Autodesk Inventor part; units mm, degrees
ref_plane "YZ Plane" through (0, 0, 0) normal (1, 0, 0) x (0, 1, 0)
ref_plane "XZ Plane" through (0, 0, 0) normal (0, 1, 0) x (-1, 0, 0)
ref_plane "XY Plane" through (0, 0, 0) normal (0, 0, 1) x (1, 0, 0)
sketch "Sketch1" plane through (0, 0, 0) normal (0, 0, 1) x (1, 0, 0)
  line L0 (-81.3375, 50) -> (81.3375, 50)
  line L1 (81.3375, 50) -> (81.3375, -50)
  line L2 (81.3375, -50) -> (-81.3375, -50)
  line L3 (-81.3375, -50) -> (-81.3375, 50)
  point P0 (0, 0)
  point P1 (0, 50)
  point P2 (81.3375, 0)
  dimension "d0" = 100
  dimension "d1" = 162.675
extrude "Extrusion1" add sketch "Sketch1" along normal blind 10
sketch "Sketch2" plane through (0, 0, 10) normal (0, 0, 1) x (1, 0, 0)
  line L0 (10.6002, 14) -> (68.6002, 14) construction
  line L1 (68.6002, 14) -> (68.6002, -35) construction
  line L2 (68.6002, -35) -> (10.6002, -35) construction
  line L3 (10.6002, -35) -> (10.6002, 14) construction
  line L4 (-81.3375, -50) -> (81.3375, -50)
  point P0 (0, 0)
  dimension "d4" = 58
  dimension "d5" = 49
  dimension "d18" = 15
hole "Hole1" at (10.6002, 14, 10) at (68.6002, 14, 10) at (68.6002, -35, 10) at (10.6002, -35, 10) direction (0, 0, -1) diameter 3 end through all
sketch "Sketch3" plane through (0, 0, 10) normal (0, 0, 1) x (1, 0, 0)
  line L0 (14.1002, -32.35) -> (65.1002, -32.35)
  line L1 (65.1002, -32.35) -> (65.1002, -37.65)
  line L2 (65.1002, -37.65) -> (14.1002, -37.65)
  line L3 (14.1002, -37.65) -> (14.1002, -32.35)
  circle A0 centre (68.6002, -35) radius 1.5
  circle A1 centre (10.6002, -35) radius 1.5
  line L4 (10.6002, -35) -> (68.6002, -35) construction
  point P0 (0, 0)
  point P1 (65.1002, -35)
  point P2 (39.6002, -35)
  point P3 (39.6002, -32.35)
  dimension "d14" = 5.3
  dimension "d15" = 51
extrude "Extrusion2" cut sketch "Sketch3" against normal through all contours L0 L1 L2 L3
mirror "Mirror1" about plane through (0, 0, 0) normal (1, 0, 0) of "Hole1", "Extrusion2"
fillet "Fillet1" radius 3 4 edges at (81.3375, 50, 5) (-81.3375, 50, 5) (-81.3375, -50, 5) (81.3375, -50, 5)
equation "\"d1\" = 2.5 * width"
equation "\"hight\" = 56.21"
equation "\"width\" = 65.07"
properties part number "RasPi-Hat-outline"
Can you work these out from the model? Positions are in its coordinate system, mm. A direction names the side the tool comes from. Give positions to 0.01 mm unless a question says otherwise; leave off trailing zeros. Loops run counter-clockwise (first coordinate to the right, second up) from the corner with the lowest first, then second, coordinate; pieces in that order, holes last. Notation, with made-up numbers: (80, 46) - (100, 46) arc R9 cw to (100, 51) - close; hole circle Ø7 at (48, -37.75). An arc over 180 degrees is marked (long way). One line per item, written item: value.
(1) If we mould it in two halves opening along Y, with no side actions, what happens to faces 3 (the face through (-9.7, -33.8, 4.9)), 4 (the face through (-1, 1, 0)), 5 (the face through (80.48, 49.1, 5.07))? For each: released by +Y, released by -Y, zero draft, split by the parting line, or undercut.
Verdict:
face 3: undercut
face 4: zero draft
face 5: released by +Y
(2) I need wall thicknesses on line 1 along X through (y, z) = (14, 8); line 2 along Y through (x, z) = (48.5, 1.75). Which ranges of each line are inside material? Lowest first, please.
Verdict:
line 1: -81.34 to -70.1, -67.1 to -12.1, -9.1 to 9.1, 12.1 to 67.1, 70.1 to 81.34
line 2: -50 to -37.65, -32.35 to 50
(3) If we section it at B-B, the plane z = 1.75: State how many separate pieces and enclosed holes the cut face has, plus the area to 3 significant figures.
Verdict:
separate pieces: 1
enclosed holes: 10
area: 15,700 mm^2
(4) On a 3-axis mill with a long thin cutter (end or side, diameter ignored), from which of +Z, -Z, +X, -X, +Y, -Y can I reach the whole of each face in a straight line? I mean faces 1 (the face through (-39, -37.65, 5)), 2 (the face through (-1, 1, 10)). Say none if no direction works.
Verdict:
face 1: +Z, -Z
face 2: +Z, +X, -X, +Y, -Y
(5) If we section it at A-A, the plane x = -34: List the corners of the cut face in (y, z) for me.
Verdict:
outline: (-50, 0) - (-37.65, 0) - (-37.65, 10) - (-50, 10) - close; (-32.35, 0) - (50, 0) - (50, 10) - (-32.35, 10) - close
(6) I'm going to push flat-ended pins straight in: pin 1 (3 mm diameter, centred on x = 41.5, y = -29.5, fed in from -Z); pin 2 (2.5 mm diameter, centred on x = -10.6, y = 14, fed in from +Z). Where does each tip first touch, or does it pass through?
Verdict:
pin 1: z = 0
pin 2: through
